Verification items for the finished model (mm, model axes). A direction names the side the tool comes from. Coordinates: 2 decimals unless noted, no trailing zeros. Write each loop counter-clockwise with the first axis right and the second up, starting at its lowest first coordinate (ties: lowest second). Pieces come first, ordered by that corner, then holes. Notation, with made-up numbers: (54.25, 35) -> (72.25, 35) arc R34 cw to (72.25, 69) -> close; hole circle Ø7 at (43, 88.25). An arc over 180 degrees is marked (long way). Answer in a Markdown table with one row per item.
```python
from build123d import *

# Parameters (mm, degrees)
F1_DEPTH = 2.5
F2_R     = 0.85
F3_DEPTH = 12.5


with BuildPart() as f1:
    # F0 (on Top) → F1 (new body)
    with BuildSketch(Plane.XY):
        with BuildLine():
            Line((13.081475452, -13.081475452), (1.0606601718, -1.0606601718))
            ThreePointArc((1.0606601718, -1.0606601718), (0, -0.6213203436), (-1.0606601718, -1.0606601718))
            Line((-1.0606601718, -1.0606601718), (-13.081475452, -13.081475452))
            ThreePointArc((-13.081475452, -13.081475452), (-13.5208152802, -14.1421356237), (-13.081475452, -15.2027957955))
            Line((-13.081475452, -15.2027957955), (-1.0606601718, -27.2236110757))
            ThreePointArc((-1.0606601718, -27.2236110757), (0, -27.6629509039), (1.0606601718, -27.2236110757))
            Line((1.0606601718, -27.2236110757), (13.081475452, -15.2027957955))
            ThreePointArc((13.081475452, -15.2027957955), (13.5208152802, -14.1421356237), (13.081475452, -13.081475452))
        make_face()
        with BuildLine():
            add(Edge.make_bspline(
                [(-2.9727151348, -10.1835160413), (-2.6797463848, -10.5025264579), (-2.6797463848, -11.0103389579)],
                knots=[0, 0, 0, 1, 1, 1], degree=2))
            add(Edge.make_bspline(
                [(-2.6797463848, -11.0103389579), (-2.6797463848, -11.6646358329), (-3.1544642668, -12.0313893052)],
                knots=[0, 0, 0, 1, 1, 1], degree=2))
            add(Edge.make_bspline(
                [(-3.1544642668, -12.0313893052), (-3.6291821487, -12.3981427774), (-4.4429842321, -12.3981427774)],
                knots=[0, 0, 0, 1, 1, 1], degree=2))
            add(Edge.make_bspline(
                [(-4.4429842321, -12.3981427774), (-5.3240606209, -12.3981427774), (-5.7993210376, -12.170278194)],
                knots=[0, 0, 0, 1, 1, 1], degree=2))
            Line((-5.7993210376, -12.170278194), (-5.7993210376, -11.6147226385))
            add(Edge.make_bspline(
                [(-5.7993210376, -11.6147226385), (-5.4933314543, -11.7427608329), (-5.1341734682, -11.8176306246)],
                knots=[0, 0, 0, 1, 1, 1], degree=2))
            add(Edge.make_bspline(
                [(-5.1341734682, -11.8176306246), (-4.7750154821, -11.8925004163), (-4.4223679126, -11.8925004163)],
                knots=[0, 0, 0, 1, 1, 1], degree=2))
            add(Edge.make_bspline(
                [(-4.4223679126, -11.8925004163), (-3.8461960376, -11.8925004163), (-3.5543123571, -11.6738589232)],
                knots=[0, 0, 0, 1, 1, 1], degree=2))
            add(Edge.make_bspline(
                [(-3.5543123571, -11.6738589232), (-3.2624286765, -11.4552174302), (-3.2624286765, -11.0645924302)],
                knots=[0, 0, 0, 1, 1, 1], degree=2))
            add(Edge.make_bspline(
                [(-3.2624286765, -11.0645924302), (-3.2624286765, -10.8074309718), (-3.3660528084, -10.643042951)],
                knots=[0, 0, 0, 1, 1, 1], degree=2))
            add(Edge.make_bspline(
                [(-3.3660528084, -10.643042951), (-3.4696769404, -10.4786549302), (-3.7121899612, -10.3392235065)],
                knots=[0, 0, 0, 1, 1, 1], degree=2))
            add(Edge.make_bspline(
                [(-3.7121899612, -10.3392235065), (-3.9547029821, -10.1997920829), (-4.4494946487, -10.0240108329)],
                knots=[0, 0, 0, 1, 1, 1], degree=2))
            add(Edge.make_bspline(
                [(-4.4494946487, -10.0240108329), (-5.1406838848, -9.7766149996), (-5.4374503779, -9.4375307982)],
                knots=[0, 0, 0, 1, 1, 1], degree=2))
            add(Edge.make_bspline(
                [(-5.4374503779, -9.4375307982), (-5.7342168709, -9.0984465968), (-5.7342168709, -8.5526566663)],
                knots=[0, 0, 0, 1, 1, 1], degree=2))
            add(Edge.make_bspline(
                [(-5.7342168709, -8.5526566663), (-5.7342168709, -7.9797399996), (-5.3039868362, -7.6406557982)],
                knots=[0, 0, 0, 1, 1, 1], degree=2))
            add(Edge.make_bspline(
                [(-5.3039868362, -7.6406557982), (-4.8737568015, -7.3015715968), (-4.1641213848, -7.3015715968)],
                knots=[0, 0, 0, 1, 1, 1], degree=2))
            add(Edge.make_bspline(
                [(-4.1641213848, -7.3015715968), (-3.4251890932, -7.3015715968), (-2.8045293709, -7.5728389579)],
                knots=[0, 0, 0, 1, 1, 1], degree=2))
            Line((-2.8045293709, -7.5728389579), (-2.9846508987, -8.0741410413))
            add(Edge.make_bspline(
                [(-2.9846508987, -8.0741410413), (-3.5988002043, -7.8169795829), (-4.1782272876, -7.8169795829)],
                knots=[0, 0, 0, 1, 1, 1], degree=2))
            add(Edge.make_bspline(
                [(-4.1782272876, -7.8169795829), (-4.6361265932, -7.8169795829), (-4.8938305862, -8.0133771524)],
                knots=[0, 0, 0, 1, 1, 1], degree=2))
            add(Edge.make_bspline(
                [(-4.8938305862, -8.0133771524), (-5.1515345793, -8.2097747218), (-5.1515345793, -8.5591670829)],
                knots=[0, 0, 0, 1, 1, 1], degree=2))
            add(Edge.make_bspline(
                [(-5.1515345793, -8.5591670829), (-5.1515345793, -8.8163285413), (-5.0565910029, -8.9812590968)],
                knots=[0, 0, 0, 1, 1, 1], degree=2))
            add(Edge.make_bspline(
                [(-5.0565910029, -8.9812590968), (-4.9616474265, -9.1461896524), (-4.7359529821, -9.2834509371)],
                knots=[0, 0, 0, 1, 1, 1], degree=2))
            add(Edge.make_bspline(
                [(-4.7359529821, -9.2834509371), (-4.5102585376, -9.4207122218), (-4.0458488154, -9.5867278468)],
                knots=[0, 0, 0, 1, 1, 1], degree=2))
            add(Edge.make_bspline(
                [(-4.0458488154, -9.5867278468), (-3.2656838848, -9.8645056246), (-2.9727151348, -10.1835160413)],
                knots=[0, 0, 0, 1, 1, 1], degree=2))
        make_face(mode=Mode.SUBTRACT)
        with BuildLine():
            Line((-8.1334756687, -14.8039748892), (-8.1334756687, -13.4802963582))
            Line((-8.1334756687, -13.4802963582), (-0.6236797201, -13.4802963582))
            Line((-0.6236797201, -13.4802963582), (-0.6236797201, -6.9198086858))
            ThreePointArc((-0.6236797201, -6.9198086858), (-0.9032194318, -6.4583786209), (-0.9135835525, -5.9189782686))
            ThreePointArc((-0.9135835525, -5.9189782686), (0.0168397474, -5.0141534426), (0.9868078824, -5.876451129))
            ThreePointArc((0.9868078824, -5.876451129), (0.9900106564, -6.4384308628), (0.6999988109, -6.9198086858))
            Line((0.6999988109, -6.9198086858), (0.6999988109, -13.4802963582))
            Line((0.6999988109, -13.4802963582), (8.1334756687, -13.4802963582))
            ThreePointArc((8.1334756687, -13.4802963582), (8.5949057336, -13.2007566465), (9.134306086, -13.1903925258))
            ThreePointArc((9.134306086, -13.1903925258), (10.0391309119, -14.1208158258), (9.1768332255, -15.0907839607))
            ThreePointArc((9.1768332255, -15.0907839607), (8.6148534917, -15.0939867347), (8.1334756687, -14.8039748892))
            Line((8.1334756687, -14.8039748892), (0.6999988109, -14.8039748892))
            Line((0.6999988109, -14.8039748892), (0.6999988109, -23.1867600232))
            Line((0.6999988109, -23.1867600232), (-0.6236797201, -23.1867600232))
            Line((-0.6236797201, -23.1867600232), (-0.6236797201, -14.8039748892))
            Line((-0.6236797201, -14.8039748892), (-8.1334756687, -14.8039748892))
        make_face(mode=Mode.SUBTRACT)
        with BuildLine():
            add(Edge.make_bspline(
                [(3.4079297135, -12.4389777291), (3.0824088802, -12.7932529027), (2.471514783, -12.7932529027)],
                knots=[0, 0, 0, 1, 1, 1], degree=2))
            add(Edge.make_bspline(
                [(2.471514783, -12.7932529027), (2.1535894357, -12.7932529027), (1.9702126996, -12.7021070694)],
                knots=[0, 0, 0, 1, 1, 1], degree=2))
            Line((1.9702126996, -12.7021070694), (1.9702126996, -12.2105706111))
            add(Edge.make_bspline(
                [(1.9702126996, -12.2105706111), (2.2110981163, -12.2778449166), (2.471514783, -12.2778449166)],
                knots=[0, 0, 0, 1, 1, 1], degree=2))
            add(Edge.make_bspline(
                [(2.471514783, -12.2778449166), (2.8078863107, -12.2778449166), (2.9825824913, -12.0743943958)],
                knots=[0, 0, 0, 1, 1, 1], degree=2))
            add(Edge.make_bspline(
                [(2.9825824913, -12.0743943958), (3.1572786719, -11.8709438749), (3.1572786719, -11.4879143611)],
                knots=[0, 0, 0, 1, 1, 1], degree=2))
            Line((3.1572786719, -11.4879143611), (3.1572786719, -6.5302320694))
            Line((3.1572786719, -6.5302320694), (3.7334505469, -6.5302320694))
            Line((3.7334505469, -6.5302320694), (3.7334505469, -11.4401713055))
            add(Edge.make_bspline(
                [(3.7334505469, -11.4401713055), (3.7334505469, -12.0847025555), (3.4079297135, -12.4389777291)],
                knots=[0, 0, 0, 1, 1, 1], degree=2))
        make_face(mode=Mode.SUBTRACT)
    extrude(amount=F1_DEPTH)

    # F2 (on Right) → F3 (cut, symmetric)
    with BuildSketch(Plane.YZ):
        with Locations((-2.4908210296, 1.292226194)):
            Circle(F2_R)
    extrude(amount=F3_DEPTH, both=True, mode=Mode.SUBTRACT)


solid = f1.part
```
1. Sectioned sample at C-C, the plane z = 0.8. Count the separate pieces of the cut face and the enclosed holes in it, and give its area (3 significant figures).
Findings below:
| item | result |
|---|---|
| separate pieces | 2 |
| enclosed holes | 3 |
| area | 334 mm² |
2. Material ranges on probe 1 along Y at (x, z) = (-4.5, 0.8); probe 2 along Y at (x, z) = (-5, 2.25); probe 3 along Y at (x, z) = (-5.5, 0.7), recorded low to high. Write a range as from..to.
Findings below:
| item | result |
|---|---|
| probe 1 | y = -23.78..-14.8, -13.48..-12.4, -11.89..-10.01, -9.41..-7.85, -7.32..-4.5 |
| probe 2 | y = -23.28..-14.8, -13.48..-12.37, -11.84..-9.78, -9.06..-8.11, -7.46..-5 |
| probe 3 | y = -22.78..-14.8, -13.48..-12.28, -11.72..-9.36, -7.83..-5.5 |
3. Sectioned sample at A-A, the plane y = -19.5. Record the cut outline in (x, z).
Findings below:
| item | result |
|---|---|
| outline | (-8.78, 0) -> (-0.62, 0) -> (-0.62, 2.5) -> (-8.78, 2.5) -> close; (0.7, 0) -> (8.78, 0) -> (8.78, 2.5) -> (0.7, 2.5) -> close |
4. Go/stop test with flat-tipped pins: pin 1 (0.8 mm diameter, centred on y = -11, z = 1, fed in from -X); pin 2 (0.8 mm diameter, centred on y = -9.5, z = 1.5, fed in from +X); pin 3 (1.2 mm diameter, centred on x = -5, z = 1.5, fed in from -Y). Record where each tip stops, or that it passes through.
Findings below:
| item | result |
|---|---|
| pin 1 | stops at x = -11.4 |
| pin 2 | stops at x = 9.9 |
| pin 3 | stops at y = -23.88 |
5. Access from +Z, -Z, +X, -X, +Y, -Y to the whole of each face (thin tool, end or side, straight path). Record for faces 1 (the face through (-13.52, -14.13, 1.23)), 2 (the face through (10.04, -14.1, 1.23)).
Findings below:
| item | result |
|---|---|
| face 1 | +Z, -Z, -X |
| face 2 | +Z, -Z |
6. Sectioned sample at B-B, the plane x = 9.5. Record the cut outline in (y, z).
Findings below:
| item | result |
|---|---|
| outline | (-18.78, 0) -> (-15, 0) -> (-15, 2.5) -> (-18.78, 2.5) -> close; (-13.28, 0) -> (-9.5, 0) -> (-9.5, 2.5) -> (-13.28, 2.5) -> close |
7. Release check for a two-part mould opening along Y. For faces 3 (the face through (0.02, -0.62, 1.23)), 4 (the face through (-0.016, -27.663, 1.232)), 5 (the face through (-0.9, -6.47, 1.23)) record: released by +Y, released by -Y, zero draft, split by the parting line, or undercut.
Findings below:
| item | result |
|---|---|
| face 3 | released by +Y |
| face 4 | released by -Y |
| face 5 | undercut |
